Geometry: final body of the model. Coordinates: model frame, mm. A direction names the side the tool comes from. Give positions to 0.01 mm unless a question says otherwise; leave off trailing zeros. Loops run counter-clockwise (first coordinate to the right, second up) from the corner with the lowest first, then second, coordinate; pieces in that order, holes last. Notation, with made-up numbers: (45, 85.5) - (56, 85.5) arc R24 ccw to (56, 95.5) - close; hole circle Ø5 at (52.25, -10). An arc over 180 degrees is marked (long way). Answer in a Markdown table with one row per item.
from build123d import *

# Parameters (mm, degrees)
F1_DEPTH  = 9.525
F2_W      = 12.7
F2_H      = 9.525
F2_W_2    = 203.2
F3_DEPTH  = 9.525
F5_DEPTH  = 114.3
F7_DEPTH  = 9.652
F8_DEPTH  = 25.4
F9_W      = 12.7
F9_H      = 76.2
F10_DEPTH = 88.9
F12_DEPTH = 25.4


with BuildPart() as f1:
    # F0 (on Front) → F1 (new body)
    with BuildSketch(Plane.XZ):
        with BuildLine():
            Line((100.1874667764, 17.9892315423), (-103.0125332236, 17.9892315423))
            Line((-103.0125332236, 17.9892315423), (-103.0125332236, -45.5107684577))
            ThreePointArc((-103.0125332236, -45.5107684577), (-94.0322771026, -49.2305123366), (-90.3125332236, -58.2107684577))
            Line((-90.3125332236, -58.2107684577), (-14.1125332236, -58.2107684577))
            ThreePointArc((-14.1125332236, -58.2107684577), (-1.4125332236, -70.9107684577), (11.2874667764, -58.2107684577))
            Line((11.2874667764, -58.2107684577), (87.4874667764, -58.2107684577))
            ThreePointArc((87.4874667764, -58.2107684577), (91.2072106553, -49.2305123366), (100.1874667764, -45.5107684577))
            Line((100.1874667764, -45.5107684577), (100.1874667764, 17.9892315423))
        make_face()
    extrude(amount=F1_DEPTH)

    # F2 (on face) → F3 (join)
    with BuildSketch(Plane.XY.offset(17.9892315423)):
        with Locations((-109.3625332236, -4.7625)):
            Rectangle(F2_W, F2_H)
        with Locations((-1.4125332236, -4.7625)):
            Rectangle(F2_W_2, F2_H)
        with Locations((106.5374667764, -4.7625)):
            Rectangle(F2_W, F2_H)
    extrude(amount=F3_DEPTH)

    # F4 (on face) → F5 (join)
    with BuildSketch(Plane.XZ.offset(9.525)):
        Polygon((-115.7125332236, 17.9892315423), (-103.0125332236, 17.9892315423), (100.1874667764, 17.9892315423), (112.8874667764, 17.9892315423), (112.8874667764, 27.5142315423), (-115.7125332236, 27.5142315423), align=None)
    extrude(amount=F5_DEPTH)

    # F6 (on face) → F7 (cut)
    with BuildSketch(Plane.XY.offset(27.5142315423)):
        with BuildLine():
            ThreePointArc((-90.3125332236, -123.825), (-108.2730454658, -116.3855122421), (-115.7125332236, -98.425))
            Line((-115.7125332236, -98.425), (-115.7125332236, -123.825))
            Line((-115.7125332236, -123.825), (-90.3125332236, -123.825))
        make_face()
    extrude(amount=-F7_DEPTH, mode=Mode.SUBTRACT)

    # F6 (on face) → F8 (cut)
    with BuildSketch(Plane.XY.offset(27.5142315423)):
        with BuildLine():
            Line((112.8874667764, -123.825), (112.8874667764, -98.425))
            ThreePointArc((112.8874667764, -98.425), (105.4479790185, -116.3855122421), (87.4874667764, -123.825))
            Line((87.4874667764, -123.825), (112.8874667764, -123.825))
        make_face()
    extrude(amount=-F8_DEPTH, mode=Mode.SUBTRACT)

    # F9 (on face) → F10 (join)
    with BuildSketch(Plane.XZ.offset(9.525)):
        with Locations((-1.4125332236, -20.1107684577)):
            Rectangle(F9_W, F9_H)
    extrude(amount=F10_DEPTH)

    # F11 (on face) → F12 (cut)
    with BuildSketch(Plane.YZ.offset(4.9374667764)):
        with BuildLine():
            ThreePointArc((-29.1272475292, -58.2107684577), (-50.2201883101, -11.5676739355), (-98.425, 5.659820001))
            Line((-98.425, 5.659820001), (-98.425, 5.2892315423))
            Line((-98.425, 5.2892315423), (-98.425, -58.2107684577))
            Line((-98.425, -58.2107684577), (-29.1272475292, -58.2107684577))
        make_face()
    extrude(amount=-F12_DEPTH, mode=Mode.SUBTRACT)


solid = f1.part
Q1. Reachability of faces 1 (the flat face through (-103.013, -5, -13)), 2 (the flat face through (-7.763, -34, -12)), 3 (the flat face through (4.937, -34, -12)), 4 (the flat face through (100.187, -5, -14)) from +Z, -Z, +X, -X, +Y, -Y: full face, straight path, thin tool, end or side. Return the list, or none.
Check values:
| item | result |
|---|---|
| face 1 | -Z, -X, +Y, -Y |
| face 2 | -Z, -X, -Y |
| face 3 | -Z, +X, -Y |
| face 4 | -Z, +X, +Y, -Y |
Q2. Cut plane B-B (z = -16). Output: boundary loops of the cut face in (x, y) (3 decimals).
Check values:
| item | result |
|---|---|
| outline | (-103.013, -9.525) - (-7.763, -9.525) - (-7.763, -45.848) - (4.937, -45.848) - (4.937, -9.525) - (100.187, -9.525) - (100.187, 0) - (-103.013, 0) - close |
Q3. Material intervals for line 1 along Y through (x, z) = (84, 9) (3 decimals); line 2 along Z through (x, y) = (57, -43.5); line 3 along X through (y, z) = (-22.5, 11), sorted ascending.
Check values:
| item | result |
|---|---|
| line 1 | -9.525 to 0 |
| line 2 | 17.99 to 27.51 |
| line 3 | -7.76 to 4.94 |
Q4. First-contact query: pin 1 (1.5 mm diameter, centred on y = -41, z = -23.5, fed in from -X); pin 2 (7.5 mm diameter, centred on x = 44.5, y = -5, fed in from -Z); pin 3 (7.5 mm diameter, centred on y = -4, z = -1.5, fed in from +X); pin 4 (10 mm diameter, centred on x = -3.5, z = 13.5, fed in from -Y) (3 decimals). Flat tips, straight axial feed; report the tip coordinate or a pass-through.
Check values:
| item | result |
|---|---|
| pin 1 | through |
| pin 2 | z = -58.21 |
| pin 3 | x = 100.19 |
| pin 4 | y = -123.825 |
Q5. Cut plane C-C (x = 84). Output: boundary loops of the cut face in (y, z) (3 decimals).
Check values:
| item | result |
|---|---|
| outline | (-123.825, 17.989) - (-9.525, 17.989) - (-9.525, -58.211) - (0, -58.211) - (0, 27.514) - (-123.825, 27.514) - close |
Q6. Cut plane A-A (y = -13). Output: boundary loops of the cut face in (x, z).
Check values:
| item | result |
|---|---|
| outline | (-115.71, 17.99) - (-7.76, 17.99) - (-7.76, -58.21) - (4.94, -58.21) - (4.94, 17.99) - (112.89, 17.99) - (112.89, 27.51) - (-115.71, 27.51) - close |
Q7. Cut plane D-D (x = -99). Output: boundary loops of the cut face in (y, z) (3 decimals).
Check values:
| item | result |
|---|---|
| outline | (-122.293, 17.989) - (-9.525, 17.989) - (-9.525, -46.161) - (0, -46.161) - (0, 27.514) - (-122.293, 27.514) - close |
